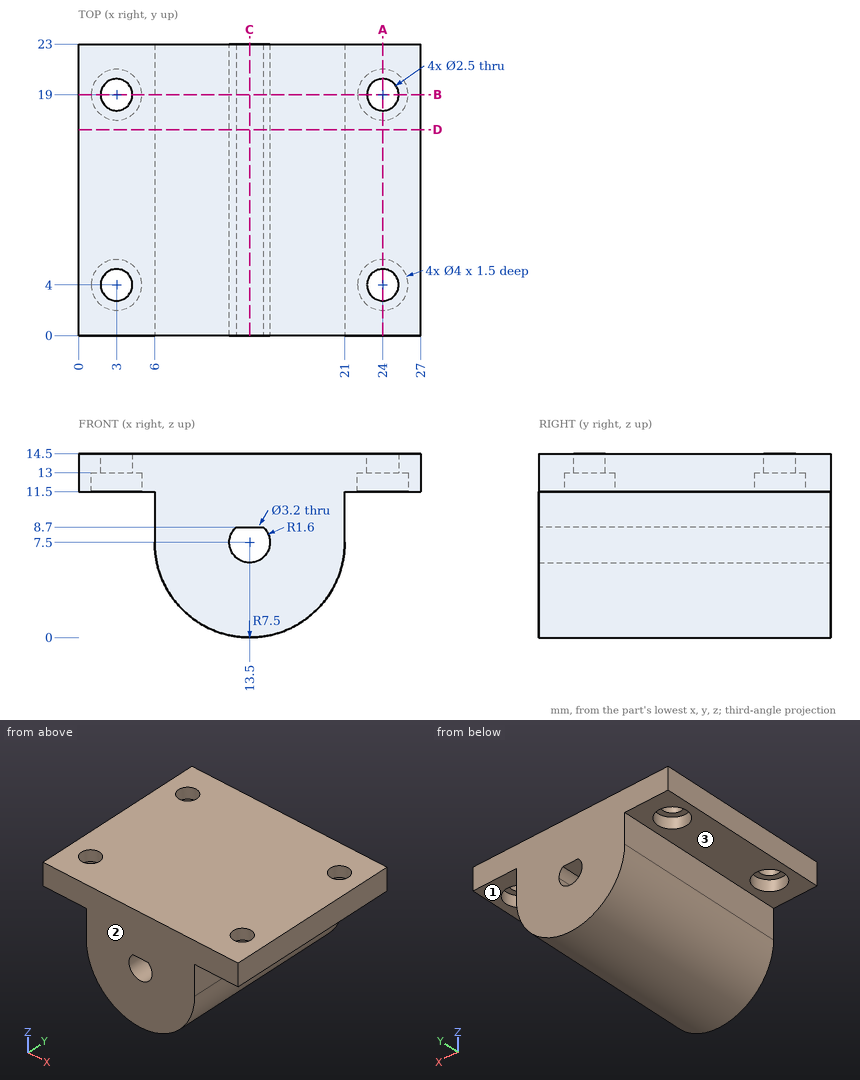
Drawing for the job (mm, zero at the part's lowest x, y, z). A direction names the side the tool comes from. Coordinates: 2 decimals unless noted, no trailing zeros. Order: outer loops, then holes, each group sorted by start corner. A loop starts at its lowest first (then second) coordinate and runs counter-clockwise, first axis right, second up. Notation, with made-up numbers: (58, 52.25) -> (78, 52.25) arc R16 cw to (78, 76.25) -> close; hole circle Ø1 at (63, 54). An arc over 180 degrees is marked (long way). One line per item, written item: value.
(1) Drop flat-ended pins along their axis: pin 1 Ø1.8 at (x, y) = (2, 12) entering from -Z; pin 2 Ø3.5 at (x, y) = (24, 4) entering from -Z; pin 3 Ø1.2 at (y, z) = (6.5, 9.5) entering from -X. Give the stop position or say it passes through.
Checked values:
pin 1: z = 11.5
pin 2: z = 13
pin 3: x = 6
(2) Slice it at D-D, the plane y = 16.25. List the corners of the cut face in (x, z).
Checked values:
outline: (0, 11.5) -> (6, 11.5) -> (6, 7.5) arc R7.5 ccw to (21, 7.5) -> (21, 11.5) -> (27, 11.5) -> (27, 14.5) -> (0, 14.5) -> close; hole (12.44, 8.7) arc R1.6 ccw (long way) to (14.56, 8.7) -> close
(3) Slice it at A-A, the plane x = 24. List the corners of the cut face in (y, z), plus the area to 3 significant figures.
Checked values:
outline: (0, 11.5) -> (2, 11.5) -> (2, 13) -> (2.75, 13) -> (2.75, 14.5) -> (0, 14.5) -> close; (5.25, 13) -> (6, 13) -> (6, 11.5) -> (17, 11.5) -> (17, 13) -> (17.75, 13) -> (17.75, 14.5) -> (5.25, 14.5) -> close; (20.25, 13) -> (21, 13) -> (21, 11.5) -> (23, 11.5) -> (23, 14.5) -> (20.25, 14.5) -> close
area: 49.5 mm2
(4) Probe line 1 (X direction, y = 4, z = 12.4); line 2 (X direction, y = 14, z = 7.5); line 3 (Y direction, x = 2.25, z = 12.5). List the from-to ranges inside material, lowest first. Write a range as [from, to].
Checked values:
line 1: [0, 1], [5, 22], [26, 27]
line 2: [6, 11.9], [15.1, 21]
line 3: [0, 2.15], [5.85, 17.15], [20.85, 23]
(5) Slice it at B-B, the plane y = 19. List the corners of the cut face in (x, z), plus the area to 3 significant figures.
Checked values:
outline: (0, 11.5) -> (1, 11.5) -> (1, 13) -> (1.75, 13) -> (1.75, 14.5) -> (0, 14.5) -> close; (4.25, 13) -> (5, 13) -> (5, 11.5) -> (6, 11.5) -> (6, 7.5) arc R7.5 ccw to (21, 7.5) -> (21, 11.5) -> (22, 11.5) -> (22, 13) -> (22.75, 13) -> (22.75, 14.5) -> (4.25, 14.5) -> close; (25.25, 13) -> (26, 13) -> (26, 11.5) -> (27, 11.5) -> (27, 14.5) -> (25.25, 14.5) -> close; hole (12.44, 8.7) arc R1.6 ccw (long way) to (14.56, 8.7) -> close
area: 202 mm2
(6) Tool access for the marked faces 1, 2 and 3: list every direction of +Z, -Z, +X, -X, +Y, -Y with a clear straight run to the whole face (end or side of a thin tool).
Checked values:
face 1: -Z, +X, +Y, -Y
face 2: +Z, -Z, +X, -X, -Y
face 3: -Z, -X, +Y, -Y
(7) Slice it at C-C, the plane x = 13.5. List the corners of the cut face in (y, z), plus the area to 3 significant figures.
Checked values:
outline: (0, 0) -> (23, 0) -> (23, 5.9) -> (0, 5.9) -> close; (0, 8.7) -> (23, 8.7) -> (23, 14.5) -> (0, 14.5) -> close
area: 269 mm2
